Part model, mm, in its own coordinate system. Face numbers are marked on the shaded views. A direction names the side the tool comes from. Give positions to 0.01 mm unless a question says otherwise; leave off trailing zeros. Order: outer loops, then holes, each group sorted by start corner. A loop starts at its lowest first (then second) coordinate and runs counter-clockwise, first axis right, second up. Notation, with made-up numbers: (-29.75, -29.5) -> (15.25, -29.5) arc R31 ccw to (15.25, -4.5) -> close; hole circle Ø10 at (5, 69). An arc over 180 degrees is marked (long way). Write item = value, one per line. Start each with the question number.
(1) Saw through at A-A, the plane z = 15. List the corners of the cut face in (x, y) (3 decimals).
(2) Flat gauge pins, fed straight in: pin 1 (10.5 mm diameter, centred on y = 15, z = 15, fed in from +X); pin 2 (10 mm diameter, centred on x = 6.5, z = 23, fed in from -Y); pin 3 (9 mm diameter, centred on x = -8.5, z = 16.5, fed in from +Y); pin 4 (5 mm diameter, centred on x = 10, z = 9.5, fed in from -Y). Where does each tip first touch, or does it go through?
(3) Saw through at B-B, the plane y = 6. List the corners of the cut face in (x, z), then the cut area to 3 significant figures.
(4) Probe line 1 along X through (y, z) = (8.5, 23); line 2 along Y through (x, z) = (26.75, 15); line 3 along X through (y, z) = (-13, 5.5) (3 decimals). List the from-to ranges inside material, lowest first. Write a range as from..to.
(5) Saw through at C-C, the plane y = 18. List the corners of the cut face in (x, z).
(6) Two-plate mould, pull along X, no slides. Class the marked faces 1, 2, 3 and 4: pulls with the +X half, pulls with the -X half, needs draft (parallel to the pull), parting line crosses it, or undercut.
(7) Saw through at D-D, the plane z = 5.5. List the corners of the cut face in (x, y) (3 decimals), then the cut area to 3 significant figures.
(8) Which spindle directions (+Z, -Z, +X, -X, +Y, -Y) get a long thin tool onto all of the face, cutting with end or side? Do the marked faces 5 and 6. Say none if no direction does.
from build123d import *

# Parameters (mm, degrees)
BOSS_EXTRUDE1_DEPTH = 30
FILLET1_R           = 10
SKETCH2_R           = 4
CUT_EXTRUDE1_DEPTH  = 72.589105316
SKETCH4_W           = 40
SKETCH4_H           = 22
CUT_EXTRUDE2_DEPTH  = 50.244289009
FILLET2_R           = 10


with BuildPart() as part:
    # Sketch1 → Boss-Extrude1 (new body)
    with BuildSketch(Plane.XY):
        with BuildLine():
            Line((-15.875, 25), (-15.875, 7))
            Line((-15.875, 7), (15.875, 7))
            Line((15.875, 7), (15.875, 25))
            Line((15.875, 25), (30, 25))
            Line((30, 25), (30, 0))
            Line((30, 0), (15.875, -25))
            ThreePointArc((15.875, -25), (0, -9.125), (-15.875, -25))
            Line((-15.875, -25), (-30, 0))
            Line((-30, 0), (-30, 25))
            Line((-30, 25), (-15.875, 25))
        make_face()
    extrude(amount=BOSS_EXTRUDE1_DEPTH)

    # Fillet1
    fillet1_edges = [part.edges().sort_by_distance(p)[0] for p in [
        (-22.9375, 25, 0),
        (22.9375, 25, 0),
        (22.9375, 25, 30),
        (-22.9375, 25, 30),
    ]]
    fillet(fillet1_edges, radius=FILLET1_R)

    # Sketch2 → Cut-Extrude1 (cut, through all)
    with BuildSketch(Plane.ZY.offset(30)):
        with Locations((15, 15)):
            Circle(SKETCH2_R)
    extrude(amount=-CUT_EXTRUDE1_DEPTH, mode=Mode.SUBTRACT)

    # Sketch4 → Cut-Extrude2 (cut, through all)
    with BuildSketch(Plane.XY.offset(30)):
        with Locations((0, 14)):
            Rectangle(SKETCH4_W, SKETCH4_H)
    extrude(amount=-CUT_EXTRUDE2_DEPTH, mode=Mode.SUBTRACT)

    # Fillet2
    fillet2_edges = [part.edges().sort_by_distance(p)[0] for p in [
        (-30, 0, 15),
        (30, 0, 15),
    ]]
    fillet(fillet2_edges, radius=FILLET2_R)


solid = part.part
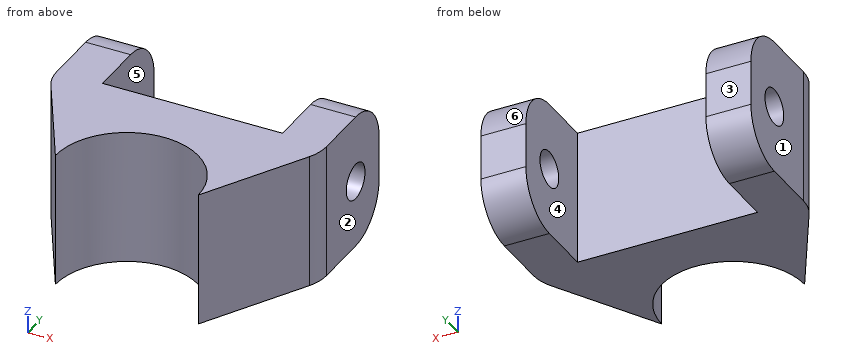
Results list:
q1.outline = (-30, 2.63) arc R10 ccw to (-28.706, -2.289) -> (-15.875, -25) arc R15.875 cw to (15.875, -25) -> (28.706, -2.289) arc R10 ccw to (30, 2.63) -> (30, 11) -> (20, 11) -> (20, 3) -> (-20, 3) -> (-20, 11) -> (-30, 11) -> close; (-30, 19) -> (-20, 19) -> (-20, 25) -> (-30, 25) -> close; (20, 19) -> (30, 19) -> (30, 25) -> (20, 25) -> close
q2.pin_1 = 30
q2.pin_2 = -14.06
q2.pin_3 = 3
q2.pin_4 = -15.21
q3.outline = (-30, 0) -> (-20, 0) -> (-20, 30) -> (-30, 30) -> close; (20, 0) -> (30, 0) -> (30, 30) -> (20, 30) -> close
q3.area = 600 mm^2
q4.line_1 = -30..-20, 20..30
q4.line_2 = -5.75..11, 19..25
q4.line_3 = -22.655..-10.393, 10.393..22.655
q5.outline = (-30, 0.46) -> (-20, 0.46) -> (-20, 12.35) -> (-30, 12.35) -> close; (-30, 17.65) -> (-20, 17.65) -> (-20, 29.54) -> (-30, 29.54) -> close; (20, 0.46) -> (30, 0.46) -> (30, 12.35) -> (20, 12.35) -> close; (20, 17.65) -> (30, 17.65) -> (30, 29.54) -> (20, 29.54) -> close
q6.face_1 = pulls with the -X half
q6.face_2 = pulls with the +X half
q6.face_3 = needs draft
q6.face_4 = undercut
q7.outline = (-30, 2.63) arc R10 ccw to (-28.706, -2.289) -> (-15.875, -25) arc R15.875 cw to (15.875, -25) -> (28.706, -2.289) arc R10 ccw to (30, 2.63) -> (30, 23.93) -> (20, 23.93) -> (20, 3) -> (-20, 3) -> (-20, 23.93) -> (-30, 23.93) -> close
q7.area = 1,350 mm^2
q8.face_5 = +Z, -Z, +Y
q8.face_6 = +Z, +X, -X, +Y
